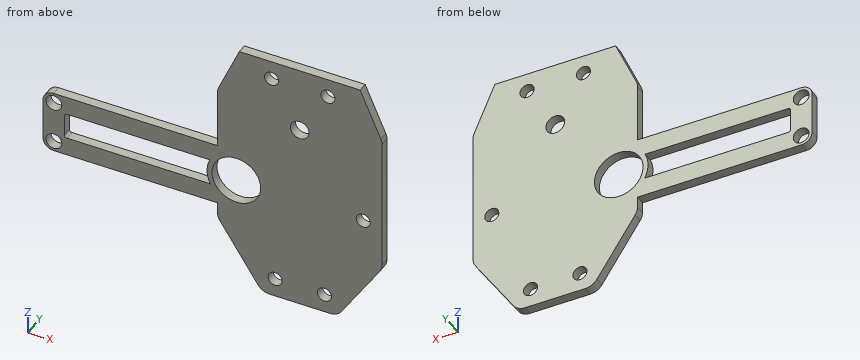
from build123d import *

# Parameters (mm, degrees)
CROQUIS1_R              = 1.5
CROQUIS1_R_2            = 2
SALIENTE_EXTRUIR1_DEPTH = 1
REDONDEO1_R             = 3
SCALE1_SCALE            = 0.888888889
SKETCH1_R               = 1.5
BOSS_EXTRUDE1_DEPTH     = 1.777777778
BOSS_EXTRUDE2_DEPTH     = 1.777777778
SKETCH3_R               = 4.6
CUT_EXTRUDE1_DEPTH      = 10


with BuildPart() as part:
    # Croquis1 → Saliente-Extruir1 (new, symmetric)
    with BuildSketch(Plane(origin=(0, 0, 0), x_dir=(1, 0, 0), z_dir=(0, 1, 0))):
        Polygon((-12.846620717, 7), (12.846620717, 7), (17.5, 17.599715907), (17.5, 47.599715907), (8, 62), (-8, 62), (-17.5, 47.599715907), (-17.5, 17.599715907), align=None)
        with Locations((-6, 11)):
            Circle(CROQUIS1_R, mode=Mode.SUBTRACT)
        with Locations((6, 11)):
            Circle(CROQUIS1_R, mode=Mode.SUBTRACT)
        with Locations((0, 21)):
            Circle(CROQUIS1_R_2, mode=Mode.SUBTRACT)
        with Locations((-13.5, 37.599715907)):
            Circle(CROQUIS1_R, mode=Mode.SUBTRACT)
        with Locations((-5.25, 57.994261746)):
            Circle(CROQUIS1_R, mode=Mode.SUBTRACT)
        with Locations((13.5, 37.599715907)):
            Circle(CROQUIS1_R, mode=Mode.SUBTRACT)
        with Locations((5.25, 57.994261746)):
            Circle(CROQUIS1_R, mode=Mode.SUBTRACT)
    extrude(amount=SALIENTE_EXTRUIR1_DEPTH, both=True)

    # Redondeo1
    redondeo1_edges = [part.edges().sort_by_distance(p)[0] for p in [
        (17.5, 0, -17.599715907),
        (-17.5, 0, -17.599715907),
        (-17.5, 0, -47.599715907),
        (-8, 0, -62),
        (8, 0, -62),
        (17.5, 0, -47.599715907),
    ]]
    fillet(redondeo1_edges, radius=REDONDEO1_R)


with BuildPart() as part_1:
    # Scale1: scaled about (0, 0, -33.418377338)
    add(part.part.scale(SCALE1_SCALE).moved(Location((0, 0, -3.713153038))))

    # Sketch1 → Boss-Extrude1 (add)
    with BuildSketch(Plane.XZ.offset(0.888888889)):
        with BuildLine():
            Line((-15.555555556, -31.135122733), (-46.555555556, -31.135122733))
            ThreePointArc((-46.555555556, -31.135122733), (-47.969769118, -31.72090917), (-48.555555556, -33.135122733))
            Line((-48.555555556, -33.135122733), (-48.555555556, -41.135122733))
            ThreePointArc((-48.555555556, -41.135122733), (-47.969769118, -42.549336295), (-46.555555556, -43.135122733))
            Line((-46.555555556, -43.135122733), (-15.555555556, -43.135122733))
            Line((-15.555555556, -43.135122733), (-15.555555556, -39.635122733))
            Line((-15.555555556, -39.635122733), (-44.013890567, -39.635122733))
            ThreePointArc((-44.013890567, -39.635122733), (-44.367443957, -39.488676123), (-44.513890567, -39.135122733))
            Line((-44.513890567, -39.135122733), (-44.513890567, -35.135122733))
            ThreePointArc((-44.513890567, -35.135122733), (-44.367443957, -34.781569342), (-44.013890567, -34.635122733))
            Line((-44.013890567, -34.635122733), (-15.555555556, -34.635122733))
            Line((-15.555555556, -34.635122733), (-15.555555556, -31.135122733))
        make_face()
        with Locations(Location((-46.5, -33.135122733, 0), (0, 0, 270))):
            Circle(SKETCH1_R, mode=Mode.SUBTRACT)
        with Locations(Location((-46.5, -41.135122733, 0), (0, 0, 270))):
            Circle(SKETCH1_R, mode=Mode.SUBTRACT)
    extrude(amount=-BOSS_EXTRUDE1_DEPTH)

    # Sketch2 → Boss-Extrude2 (add)
    with BuildSketch(Plane(origin=(0, 0.888888889, 0), x_dir=(1, 0, 0), z_dir=(0, 1, 0))):
        with BuildLine():
            Line((-16.898979486, 39.635122733), (-15.555555556, 39.635122733))
            Line((-15.555555556, 39.635122733), (-15.555555556, 34.635122733))
            Line((-15.555555556, 34.635122733), (-17.0003696, 34.635122733))
            ThreePointArc((-17.0003696, 34.635122733), (-17.54520316, 37.147198875), (-16.898979486, 39.635122733))
        make_face()
    extrude(amount=-BOSS_EXTRUDE2_DEPTH)

    # Sketch3 → Cut-Extrude1 (cut)
    with BuildSketch(Plane(origin=(0, 0.888888889, 0), x_dir=(1, 0, 0), z_dir=(0, 1, 0))):
        with Locations(Location((-12, 37.135122733, 0), (0, 0, 270))):
            Circle(SKETCH3_R)
    extrude(amount=-CUT_EXTRUDE1_DEPTH, mode=Mode.SUBTRACT)


solid = part_1.part
Work out the finished part from the listing and answer in its coordinate system (mm). Round coordinates to 2 decimals unless told otherwise and drop trailing zeros. Write each loop counter-clockwise with the first axis right and the second up, starting at its lowest first coordinate (ties: lowest second). Pieces come first, ordered by that corner, then holes. Notation, with made-up numbers: M 78.5,53 L 121.5,53 A16 ccw 121.5,75 Z; hole C 9.25,59 d9. An arc over 180 degrees is marked long. Use a Markdown table: item, result.
1) The part is cut by section A-A on x = 0. Give the vertices of the cut face in (y, z), plus the area to 3 significant figures.
Taken from the geometry:
| item | result |
|---|---|
| outline | M -0.89,-58.82 L 0.89,-58.82 L 0.89,-24.16 L -0.89,-24.16 Z; M -0.89,-20.6 L 0.89,-20.6 L 0.89,-9.94 L -0.89,-9.94 Z |
| area | 80.6 mm2 |
2) Consider line 1 (X direction, y = -0.35, z = -56); line 2 (X direction, y = -0.35, z = -33); line 3 (Z direction, x = -26, y = -0.8). Determine where each line is inside the solid, lowest interval first. Write a range as [from, to].
Taken from the geometry:
| item | result |
|---|---|
| line 1 | x = [-8.97, -5.78], [-3.56, 3.56], [5.78, 8.97] |
| line 2 | x = [-48.55, -47.99], [-45.01, -14.02], [-9.98, 15.56] |
| line 3 | z = [-43.14, -39.64], [-34.64, -31.14] |
3) The part is cut by section D-D on y = 0.5. State how many separate pieces and enclosed holes the cut face has, plus the area to 3 significant figures.
Taken from the geometry:
| item | result |
|---|---|
| separate pieces | 1 |
| enclosed holes | 10 |
| area | 1,510 mm2 |
4) The part is cut by section C-C on z = -27. Give the vertices of the cut face in (x, y).
Taken from the geometry:
| item | result |
|---|---|
| outline | M -15.56,-0.89 L 15.56,-0.89 L 15.56,0.89 L -15.56,0.89 Z |
5) The part is cut by section B-B on x = -38. Give the vertices of the cut face in (y, z), plus the area to 3 significant figures.
Taken from the geometry:
| item | result |
|---|---|
| outline | M -0.89,-43.14 L 0.89,-43.14 L 0.89,-39.64 L -0.89,-39.64 Z; M -0.89,-34.64 L 0.89,-34.64 L 0.89,-31.14 L -0.89,-31.14 Z |
| area | 12.4 mm2 |
6) Flat-ended cylindrical pins translate along their axes: pin 1 (0.5 mm diameter, centred on y = 0, z = -44, fed in from -X); pin 2 (0.9 mm diameter, centred on x = -29, y = 0, fed in from +Z); pin 3 (0.5 mm diameter, centred on x = -25, y = -0.5, fed in from -Z). Find the tip coordinate at first contact, or state that the pin passes through.
Taken from the geometry:
| item | result |
|---|---|
| pin 1 | stops at x = -15.56 |
| pin 2 | stops at z = -31.14 |
| pin 3 | stops at z = -43.14 |
